```python
from build123d import *

# Parameters (mm, degrees)
SKETCH1_W           = 29.97
SKETCH1_H           = 46.6
BOSS_EXTRUDE1_DEPTH = 3
BOSS_EXTRUDE2_DEPTH = 2
FILLET1_R           = 3


with BuildPart() as part:
    # Sketch1 → Boss-Extrude1 (new body)
    with BuildSketch(Plane(origin=(0, 0, 0), x_dir=(1, 0, 0), z_dir=(0, 1, 0))):
        Rectangle(SKETCH1_W, SKETCH1_H)
    extrude(amount=BOSS_EXTRUDE1_DEPTH)

    # Sketch2 → Boss-Extrude2 (add)
    with BuildSketch(Plane(origin=(0, 3, 0), x_dir=(1, 0, 0), z_dir=(0, 1, 0))):
        Polygon((-4.5, 19), (-4.5, 20), (-11.685, 20), (-11.685, -20), (-1.5, -20), (-1.5, -19), (-10.685, -19), (-10.685, 19), align=None)
        Polygon((11.685, -20), (11.685, 20), (4.5, 20), (4.5, 19), (10.685, 19), (10.685, -19), (1.5, -19), (1.5, -20), align=None)
    extrude(amount=BOSS_EXTRUDE2_DEPTH)

    # Fillet1
    fillet1_edges = [part.edges().sort_by_distance(p)[0] for p in [
        (14.985, 1.5, -23.3),
        (14.985, 1.5, 23.3),
        (-14.985, 1.5, 23.3),
        (-14.985, 1.5, -23.3),
    ]]
    fillet(fillet1_edges, radius=FILLET1_R)


solid = part.part
```
Verification items for the finished model (mm, model axes). A direction names the side the tool comes from. Give positions to 0.01 mm unless a question says otherwise; leave off trailing zeros. Order: outer loops, then holes, each group sorted by start corner. A loop starts at its lowest first (then second) coordinate and runs counter-clockwise, first axis right, second up. Notation, with made-up numbers: (28.25, 27) -> (45.25, 27) arc R13 ccw to (45.25, 45) -> close; hole circle Ø11 at (-24.75, 74.5). An arc over 180 degrees is marked (long way). One line per item, written item: value.
(1) Sectioned sample at B-B on x = 9.5. Record the cut outline in (y, z), then the cut area to 3 significant figures.
Final values:
outline: (0, -23.3) -> (3, -23.3) -> (3, -20) -> (5, -20) -> (5, -19) -> (3, -19) -> (3, 19) -> (5, 19) -> (5, 20) -> (3, 20) -> (3, 23.3) -> (0, 23.3) -> close
area: 144 mm^2
(2) Sectioned sample at A-A on y = 3.75. Record the cut outline in (x, z) (3 decimals).
Final values:
outline: (-11.685, -20) -> (-4.5, -20) -> (-4.5, -19) -> (-10.685, -19) -> (-10.685, 19) -> (-1.5, 19) -> (-1.5, 20) -> (-11.685, 20) -> close; (1.5, 19) -> (10.685, 19) -> (10.685, -19) -> (4.5, -19) -> (4.5, -20) -> (11.685, -20) -> (11.685, 20) -> (1.5, 20) -> close
(3) Sectioned sample at C-C on z = 3. Record the cut outline in (x, y) (3 decimals), then the cut area to 3 significant figures.
Final values:
outline: (-14.985, 0) -> (14.985, 0) -> (14.985, 3) -> (11.685, 3) -> (11.685, 5) -> (10.685, 5) -> (10.685, 3) -> (-10.685, 3) -> (-10.685, 5) -> (-11.685, 5) -> (-11.685, 3) -> (-14.985, 3) -> close
area: 93.9 mm^2
(4) Sectioned sample at D-D on x = -13. Record the cut outline in (y, z), then the cut area to 3 significant figures.
Final values:
outline: (0, -23.12) -> (3, -23.12) -> (3, 23.12) -> (0, 23.12) -> close
area: 139 mm^2
(5) Gauge pin test, flat ends, axial feed: pin 1 (1 mm diameter, centred on x = 6, y = 4, fed in from -Z); pin 2 (1.1 mm diameter, centred on y = 4, z = -19.5, fed in from +X) (3 decimals); pin 3 (0.6 mm diameter, centred on x = -7, y = 4.5, fed in from +Z). Record the tip position at first contact, or that the pin passes through.
Final values:
pin 1: z = -20
pin 2: x = 11.685
pin 3: z = 20
(6) Tool access check on faces 5 (the face through (-6, 4, 19)), 6 (the face through (7, 4, 20)), 7 (the face through (-11.685, 4, 0)). Record the directions out of +Z, -Z, +X, -X, +Y, -Y that give a thin tool (end or side, any length) a straight path to the whole face; none if there is none.
Final values:
face 5: +Y
face 6: +Z, +X, -X, +Y
face 7: +Z, -Z, -X, +Y
(7) Draft check along X on faces 1 (the face through (14.083, 1.521, 22.445)), 2 (the face through (1.5, 4, 19.5)), 3 (the face through (-14.13, 1.52, 22.4)), 4 (the face through (-7, 4, 20)). Enter one of: pulls with the +X half, pulls with the -X half, needs draft (parallel to the pull), parting line crosses it, or undercut.
Final values:
face 1: pulls with the +X half
face 2: undercut
face 3: pulls with the -X half
face 4: needs draft
(8) Scan lines: line 1 along Z through (x, y) = (-7.25, 3.15); line 2 along X through (y, z) = (3.65, -10) (3 decimals); line 3 along Z through (x, y) = (-2.25, 4.2). Record each from-to range of solid material in increasing order. Write a range as [from, to].
Final values:
line 1: [-20, -19], [19, 20]
line 2: [-11.685, -10.685], [10.685, 11.685]
line 3: [19, 20]
